from build123d import *

# Parameters (mm, degrees)
F0_W     = 76.2
F0_H     = 76.2
F1_DEPTH = 2.54
F2_SIZE  = 2.53999


# Not quite as in the source:
# - a fillet or chamfer is up to 0.001 mm smaller than in the source, because OpenCascade refuses the exact size


with BuildPart() as f1:
    # F0 (on Top) → F1 (new body)
    with BuildSketch(Plane.XY):
        with Locations((38.1, 38.1)):
            Rectangle(F0_W, F0_H)
    extrude(amount=F1_DEPTH)

    # F2 (size 2.54 in the source; OpenCascade refuses exactly that, so slightly less here)
    f2_edges = [f1.edges().sort_by_distance(p)[0] for p in [
        (0, 38.1, 0),
        (38.1, 0, 0),
        (76.2, 38.1, 0),
        (38.1, 76.2, 0),
    ]]
    chamfer(f2_edges, length=F2_SIZE)


solid = f1.part
Can you work these out from the model? Positions are in its coordinate system, mm. Give positions to 0.01 mm unless a question says otherwise; leave off trailing zeros. Order: outer loops, then holes, each group sorted by start corner. A loop starts at its lowest first (then second) coordinate and runs counter-clockwise, first axis right, second up. Notation, with made-up numbers: M -28,-19.75 L -1,-19.75 A33 ccw -1,13.25 Z; hole C 63,-7.75 d1. An arc over 180 degrees is marked long. One line per question, with ' | ' between items.
Item 1: I'm going to push flat-ended pins straight in: pin 1 Ø1 at (x, z) = (41.5, 2) entering from +Y; pin 2 Ø1 at (x, z) = (51.5, 2) entering from -Y; pin 3 Ø1 at (x, z) = (61.5, 1.5) entering from +Y. Where does each tip first touch, or does it pass through?
Answer block:
pin 1: stops at y = 76.16 | pin 2: stops at y = 0.04 | pin 3: stops at y = 75.66
Item 2: Suppose I cut it at B-B, the plane z = 0.85. Write out the boundary of the cut face in (x, y), then the cut area to 3 significant figures.
Answer block:
outline: M 1.69,1.69 L 74.51,1.69 L 74.51,74.51 L 1.69,74.51 Z | area: 5,300 mm2
Item 3: Please list where these lines run through material, in increasing order: L1, parallel to Y at x = 20, z = 1.9; L2, parallel to X at y = 10, z = 0.4; L3, parallel to X at y = 25, z = 2.2.
Answer block:
L1: y = 0.64 to 75.56 | L2: x = 2.14 to 74.06 | L3: x = 0.34 to 75.86
